Design review of the part built by this model. Coordinates are the model's own, in mm. Face numbers are marked on the shaded views. A direction names the side the tool comes from. Round coordinates to 2 decimals unless told otherwise and drop trailing zeros. Write each loop counter-clockwise with the first axis right and the second up, starting at its lowest first coordinate (ties: lowest second). Pieces come first, ordered by that corner, then holes. Notation, with made-up numbers: (60.5, -12.75) -> (117.5, -12.75) arc R8 ccw to (117.5, -3.75) -> close; hole circle Ø2 at (-39, -18). An arc over 180 degrees is marked (long way). One line per question, with ' | ' between items. Start each with the question number.
1) Consider section B-B (y = -31). Give the boundary of the cut face in (x, z), then the cut area to 3 significant figures.
2) Consider section C-C (z = 0). Count the separate pieces of the cut face and the enclosed holes in it, then the cut area to 3 significant figures.
3) Consider section A-A (x = 0). Give the boundary of the cut face in (y, z).
4) For the marked faces 4, 5, 6, 7 and 8, list the 3-axis set-ups (+Z, -Z, +X, -X, +Y, -Y) from which the entire face can be reached by the end or side of a thin tool; tool diameter is ignored.
5) Mouldability with a two-part tool opening along X and no side actions: class the marked faces 1, 2 and 3 as +X half, -X half, draft (parallel to the pull), parting line (faces both ways), or undercut.
6) For probe 1 along Z at (x, y) = (0, -32); probe 2 along X at (y, z) = (-30.75, 0); probe 3 along Z at (x, y) = (30, -22), list the stretches that pass through material, from the lowest coordinate up.
7) Insertion check: pin 1 Ø8 at (y, z) = (-14.5, -7.5) entering from -X; pin 2 Ø4 at (y, z) = (-12, -6.5) entering from -X; pin 3 Ø3 at (y, z) = (-14.5, 0) entering from -X. Each pin has a flat end and moves straight along its axis. Give the tip position at first contact, or say it passes through.
8) Consider section D-D (y = -10). Give the boundary of the cut face in (x, z), then the cut area to 3 significant figures.
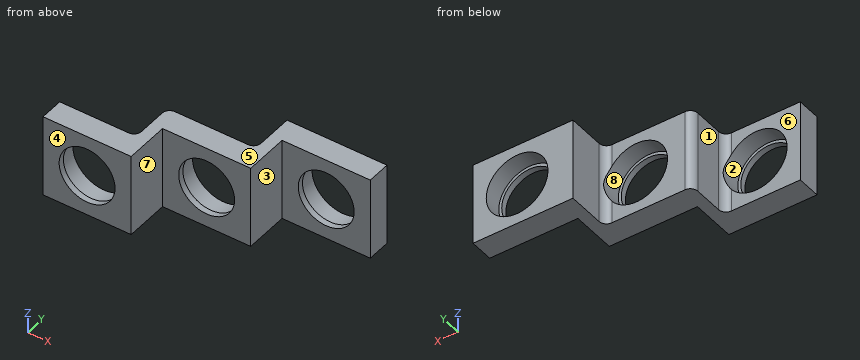
```python
from build123d import *

# Parameters (mm, degrees)
F0_W     = 30
F0_H     = 28
F0_R     = 10.5
F0_R_2   = 9.5
F1_DEPTH = 8
F2_DEPTH = 38
F3_DEPTH = 23
F4_DEPTH = 36
F5_DEPTH = 21
F6_DEPTH = 6
F8_DEPTH = 28.001


with BuildPart() as f1:
    # F0 (on Front) → F1 (new body)
    with BuildSketch(Plane.XZ):
        with Locations((60, 0)):
            Rectangle(F0_W, F0_H)
        with Locations((60, 0)):
            Circle(F0_R, mode=Mode.SUBTRACT)
        with Locations((30, 0)):
            Rectangle(F0_W, F0_H)
        with Locations((30, 0)):
            Circle(F0_R, mode=Mode.SUBTRACT)
        Rectangle(F0_W, F0_H)
        Circle(F0_R, mode=Mode.SUBTRACT)
        Circle(F0_R)
        Circle(F0_R_2, mode=Mode.SUBTRACT)
        with Locations((60, 0)):
            Circle(F0_R)
        with Locations((60, 0)):
            Circle(F0_R_2, mode=Mode.SUBTRACT)
        with Locations((30, 0)):
            Circle(F0_R)
        with Locations((30, 0)):
            Circle(F0_R_2, mode=Mode.SUBTRACT)
    extrude(amount=F1_DEPTH)

    # F0 (on Front) → F2 (join)
    with BuildSketch(Plane.XZ):
        Rectangle(F0_W, F0_H)
        Circle(F0_R, mode=Mode.SUBTRACT)
        Circle(F0_R)
        Circle(F0_R_2, mode=Mode.SUBTRACT)
    extrude(amount=F2_DEPTH)

    # F0 (on Front) → F3 (join)
    with BuildSketch(Plane.XZ):
        with Locations((30, 0)):
            Rectangle(F0_W, F0_H)
        with Locations((30, 0)):
            Circle(F0_R, mode=Mode.SUBTRACT)
        with Locations((30, 0)):
            Circle(F0_R)
        with Locations((30, 0)):
            Circle(F0_R_2, mode=Mode.SUBTRACT)
    extrude(amount=F3_DEPTH)

    # F0 (on Front) → F4 (cut)
    with BuildSketch(Plane.XZ):
        Circle(F0_R)
        Circle(F0_R_2, mode=Mode.SUBTRACT)
    extrude(amount=F4_DEPTH, mode=Mode.SUBTRACT)

    # F0 (on Front) → F5 (cut)
    with BuildSketch(Plane.XZ):
        with Locations((30, 0)):
            Circle(F0_R)
        with Locations((30, 0)):
            Circle(F0_R_2, mode=Mode.SUBTRACT)
    extrude(amount=F5_DEPTH, mode=Mode.SUBTRACT)

    # F0 (on Front) → F6 (cut)
    with BuildSketch(Plane.XZ):
        with Locations((60, 0)):
            Circle(F0_R)
        with Locations((60, 0)):
            Circle(F0_R_2, mode=Mode.SUBTRACT)
    extrude(amount=F6_DEPTH, mode=Mode.SUBTRACT)

    # F7 (on face) → F8 (cut, through all)
    with BuildSketch(Plane(origin=(0, 0, -14), x_dir=(1, 0, 0), z_dir=(0, 0, -1))):
        with BuildLine():
            Line((8.46, 30), (-15, 30))
            Line((-15, 30), (-15, 0))
            Line((-15, 0), (41, 0))
            Line((41, 0), (41, 12.46))
            ThreePointArc((41, 12.46), (40.2560512242, 14.2560512242), (38.46, 15))
            Line((38.46, 15), (13.54, 15))
            ThreePointArc((13.54, 15), (11.7439487758, 15.7439487758), (11, 17.54))
            Line((11, 17.54), (11, 27.46))
            ThreePointArc((11, 27.46), (10.2560512242, 29.2560512242), (8.46, 30))
        make_face()
    extrude(amount=-F8_DEPTH, mode=Mode.SUBTRACT)


solid = f1.part
```
From the geometry:
1) outline: (-15, -14) -> (15, -14) -> (15, 14) -> (-15, 14) -> close; hole circle Ø21 at (0, 0) | area: 494 mm2
2) separate pieces: 4 | enclosed holes: 0 | area: 348 mm2
3) outline: (-38, -14) -> (-30, -14) -> (-30, -10.5) -> (-36, -10.5) -> (-36, -9.5) -> (-38, -9.5) -> close; (-38, 9.5) -> (-36, 9.5) -> (-36, 10.5) -> (-30, 10.5) -> (-30, 14) -> (-38, 14) -> close
4) face 4: +Z, -Z, +X, -X, -Y | face 5: +Z, +X, -X, +Y, -Y | face 6: +Z, -Z, -X, +Y | face 7: +Z, -Z, +X, -Y | face 8: +Y
5) face 1: -X half | face 2: undercut | face 3: +X half
6) probe 1: z = -14 to -10.5, 10.5 to 14 | probe 2: x = -15 to -10.5, 10.5 to 15 | probe 3: z = -14 to -9.5, 9.5 to 14
7) pin 1: stops at x = 11 | pin 2: stops at x = 40.48 | pin 3: stops at x = 11.52
8) outline: (41, -14) -> (45, -14) -> (45, 14) -> (41, 14) -> close | area: 112 mm2
